from build123d import *

# Parameters (mm, degrees)
CROQUIS1_W               = 25
CROQUIS1_H               = 44
SALIENTE_EXTRUIR1_DEPTH  = 20
CROQUIS2_W               = 11.3
CROQUIS2_H               = 40.4
CORTAR_EXTRUIR1_DEPTH    = 18
CROQUIS3_W               = 10.7
CROQUIS3_H               = 44
CORTAR_EXTRUIR2_DEPTH    = 12
CORTAR_EXTRUIR3_START    = -25
CROQUIS4_R               = 1.6
CORTAR_EXTRUIR3_DEPTH    = 25
CROQUIS5_R               = 3
CORTAR_EXTRUIR4_DEPTH    = 17
CROQUIS7_W               = 10.7
CROQUIS7_H               = 2.131966011
SALIENTE_EXTRUIR2_DEPTH  = 12
CROQUIS9_W               = 11.3
CROQUIS9_H               = 12.16552506
SALIENTE_EXTRUIR3_DEPTH  = 2
SALIENTE_EXTRUIR4_DEPTH  = 2
CORTAR_EXTRUIR10_START   = -25
CROQUIS12_W              = 0.99
CROQUIS12_H              = 44
CORTAR_EXTRUIR10_DEPTH   = 25
CROQUIS13_W              = 8
CROQUIS13_H              = 44
CORTAR_EXTRUIR11_DEPTH   = 11.7
SALIENTE_EXTRUIR5_DEPTH  = 11.7
CROQUIS15_W              = 10.763613753
CROQUIS15_H              = 40.736067978
CORTAR_EXTRUIR12_DEPTH   = 4
CROQUIS16_R              = 1.5
SALIENTE_EXTRUIR6_DEPTH  = 1.2
CORTAR_EXTRUIR13_START   = -44
CORTAR_EXTRUIR13_DEPTH   = 44
CROQUIS18_W              = 0.936386247
CROQUIS18_H              = 40.568033989
CORTAR_EXTRUIR14_DEPTH   = 4
SALIENTE_EXTRUIR7_START  = -9.2
SALIENTE_EXTRUIR7_DEPTH  = 9.2
SALIENTE_EXTRUIR8_START  = -12.9
CROQUIS20_W              = 4
CROQUIS20_H              = 0.236067978
CROQUIS20_H_2            = 0.25
SALIENTE_EXTRUIR8_DEPTH  = 12.9
CROQUIS21_W              = 4
CROQUIS21_H              = 6.401046148
CROQUIS21_H_2            = 6.387114126
SALIENTE_EXTRUIR9_DEPTH  = 1.5
SALIENTE_EXTRUIR10_DEPTH = 0.4
CORTAR_EXTRUIR15_START   = -18
CROQUIS23_W              = 12.2
CROQUIS23_H              = 40.9
CORTAR_EXTRUIR15_DEPTH   = 18


with BuildPart() as part:
    # Croquis1 → Saliente-Extruir1 (new body)
    with BuildSketch(Plane.XY):
        with Locations((-22.114132301, -13.090425532)):
            Rectangle(CROQUIS1_W, CROQUIS1_H)
    extrude(amount=SALIENTE_EXTRUIR1_DEPTH)

    # Croquis2 → Cortar-Extruir1 (cut)
    with BuildSketch(Plane.XY.offset(20)):
        with Locations((-26.964132301, -13.090425532)):
            Rectangle(CROQUIS2_W, CROQUIS2_H)
    extrude(amount=-CORTAR_EXTRUIR1_DEPTH, mode=Mode.SUBTRACT)

    # Croquis3 → Cortar-Extruir2 (cut)
    with BuildSketch(Plane.XY.offset(20)):
        with Locations((-14.964132301, -13.090425532)):
            Rectangle(CROQUIS3_W, CROQUIS3_H)
    extrude(amount=-CORTAR_EXTRUIR2_DEPTH, mode=Mode.SUBTRACT)

    # Croquis4 → Cortar-Extruir3 (cut)
    with BuildSketch(Plane.ZY.offset(34.614132301).offset(CORTAR_EXTRUIR3_START)):
        with Locations((6, 2.409574468)):
            Circle(CROQUIS4_R)
        with Locations((6, -28.590425532)):
            Circle(CROQUIS4_R)
        with BuildLine():
            Line((20, 5.909574468), (20, -32.090425532))
            ThreePointArc((20, -32.090425532), (1, -13.090425532), (20, 5.909574468))
        make_face()
    extrude(amount=CORTAR_EXTRUIR3_DEPTH, mode=Mode.SUBTRACT)

    # Croquis5 → Cortar-Extruir4 (cut)
    with BuildSketch(Plane.ZY.offset(34.614132301)):
        with Locations((6, 2.409574468)):
            Circle(CROQUIS5_R)
        with Locations((6, -28.590425532)):
            Circle(CROQUIS5_R)
    extrude(amount=-CORTAR_EXTRUIR4_DEPTH, mode=Mode.SUBTRACT)

    # Croquis7 → Saliente-Extruir2 (add)
    with BuildSketch(Plane.XY.offset(8)):
        with Locations((-14.964132301, -34.024442527)):
            Rectangle(CROQUIS7_W, CROQUIS7_H)
        with Locations((-14.964132301, 7.843591463)):
            Rectangle(CROQUIS7_W, CROQUIS7_H)
    extrude(amount=SALIENTE_EXTRUIR2_DEPTH)

    # Croquis9 → Saliente-Extruir3 (add)
    with BuildSketch(Plane.XY.offset(2)):
        with Locations((-26.964132301, -13.090425532)):
            Rectangle(CROQUIS9_W, CROQUIS9_H)
    extrude(amount=-SALIENTE_EXTRUIR3_DEPTH)

    # Croquis11 → Saliente-Extruir4 (add)
    with BuildSketch(Plane.ZY.offset(32.614132301)):
        with BuildLine():
            Line((2, -7.007663002), (2, -19.173188062))
            ThreePointArc((2, -19.173188062), (1, -13.090425532), (2, -7.007663002))
        make_face()
    extrude(amount=SALIENTE_EXTRUIR4_DEPTH)

    # Croquis12 → Cortar-Extruir10 (cut)
    with BuildSketch(Plane.ZY.offset(34.614132301).offset(CORTAR_EXTRUIR10_START)):
        with Locations((0.495, -13.090425532)):
            Rectangle(CROQUIS12_W, CROQUIS12_H)
    extrude(amount=CORTAR_EXTRUIR10_DEPTH, mode=Mode.SUBTRACT)

    # Croquis13 → Cortar-Extruir11 (cut)
    with BuildSketch(Plane(origin=(-9.614132301, 0, 0), x_dir=(0, 0, -1), z_dir=(1, 0, 0))):
        with Locations((-16, -13.090425532)):
            Rectangle(CROQUIS13_W, CROQUIS13_H)
    extrude(amount=-CORTAR_EXTRUIR11_DEPTH, mode=Mode.SUBTRACT)

    # Croquis14 → Saliente-Extruir5 (add)
    with BuildSketch(Plane(origin=(-21.314132301, 0, 0), x_dir=(0, 0, -1), z_dir=(1, 0, 0))):
        with BuildLine():
            Line((-2, -19.173188062), (-2, -7.007663002))
            ThreePointArc((-2, -7.007663002), (-1, -13.090425532), (-2, -19.173188062))
        make_face()
    extrude(amount=SALIENTE_EXTRUIR5_DEPTH)

    # Croquis15 → Cortar-Extruir12 (cut)
    with BuildSketch(Plane.XY.offset(12)):
        with Locations((-14.995939178, -13.090425532)):
            Rectangle(CROQUIS15_W, CROQUIS15_H)
    extrude(amount=-CORTAR_EXTRUIR12_DEPTH, mode=Mode.SUBTRACT)

    # Croquis16 → Saliente-Extruir6 (add)
    with BuildSketch(Plane(origin=(-9.614132301, 0, 0), x_dir=(0, 0, -1), z_dir=(1, 0, 0))):
        with BuildLine():
            Line((-8, -27.821345395), (-8, -33.458459521))
            Line((-8, -33.458459521), (-12, -33.458459521))
            Line((-12, -33.458459521), (-12, -35.090425532))
            Line((-12, -35.090425532), (-0.99, -35.090425532))
            Line((-0.99, -35.090425532), (-0.99, 8.909574468))
            Line((-0.99, 8.909574468), (-12, 8.909574468))
            Line((-12, 8.909574468), (-12, 7.277608457))
            Line((-12, 7.277608457), (-8, 7.277608457))
            Line((-8, 7.277608457), (-8, 1.640494331))
            ThreePointArc((-8, 1.640494331), (-4.389181434, -2.259804881), (-2, -7.007663002))
            Line((-2, -7.007663002), (-2, -19.173188062))
            ThreePointArc((-2, -19.173188062), (-4.389181434, -23.921046183), (-8, -27.821345395))
        make_face()
        with Locations((-6, -28.590425532)):
            Circle(CROQUIS16_R, mode=Mode.SUBTRACT)
        with Locations((-6, 2.409574468)):
            Circle(CROQUIS16_R, mode=Mode.SUBTRACT)
    extrude(amount=SALIENTE_EXTRUIR6_DEPTH)

    # Croquis17 → Cortar-Extruir13 (cut)
    with BuildSketch(Plane.XZ.offset(35.090425532).offset(CORTAR_EXTRUIR13_START)):
        Polygon((-21.314132301, 12), (-21.314132301, 20), (-27.964132301, 20), align=None)
    extrude(amount=CORTAR_EXTRUIR13_DEPTH, mode=Mode.SUBTRACT)

    # Croquis18 → Cortar-Extruir14 (cut)
    with BuildSketch(Plane.XY.offset(12)):
        with Locations((-20.845939178, -13.006408538)):
            Rectangle(CROQUIS18_W, CROQUIS18_H)
    extrude(amount=-CORTAR_EXTRUIR14_DEPTH, mode=Mode.SUBTRACT)

    # Croquis19 → Saliente-Extruir7 (add)
    with BuildSketch(Plane(origin=(-8.414132301, 0, 0), x_dir=(0, 0, -1), z_dir=(1, 0, 0)).offset(SALIENTE_EXTRUIR7_START)):
        with BuildLine():
            Line((-2, -19.173188062), (-2, -7.007663002))
            ThreePointArc((-2, -7.007663002), (-4.389181434, -2.259804881), (-8, 1.640494331))
            Line((-8, 1.640494331), (-8, 0.640494331))
            ThreePointArc((-8, 0.640494331), (-5.026875227, -2.874277954), (-3, -7.007663002))
            Line((-3, -7.007663002), (-3, -19.173188062))
            ThreePointArc((-3, -19.173188062), (-4.972698099, -23.341991528), (-8, -26.821345395))
            Line((-8, -26.821345395), (-8, -27.821345395))
            ThreePointArc((-8, -27.821345395), (-4.389181434, -23.921046183), (-2, -19.173188062))
        make_face()
    extrude(amount=SALIENTE_EXTRUIR7_DEPTH)

    # Croquis20 → Saliente-Extruir8 (add)
    with BuildSketch(Plane(origin=(-8.414132301, 0, 0), x_dir=(0, 0, -1), z_dir=(1, 0, 0)).offset(SALIENTE_EXTRUIR8_START)):
        with Locations((-10, -33.340425532)):
            Rectangle(CROQUIS20_W, CROQUIS20_H)
        with Locations((-10, 7.152608457)):
            Rectangle(CROQUIS20_W, CROQUIS20_H_2)
    extrude(amount=SALIENTE_EXTRUIR8_DEPTH)

    # Croquis21 → Saliente-Extruir9 (add)
    with BuildSketch(Plane(origin=(-8.414132301, 0, 0), x_dir=(0, 0, -1), z_dir=(1, 0, 0))):
        with Locations((-10, -30.021868469)):
            Rectangle(CROQUIS21_W, CROQUIS21_H)
        with Locations((-10, 3.834051394)):
            Rectangle(CROQUIS21_W, CROQUIS21_H_2)
    extrude(amount=-SALIENTE_EXTRUIR9_DEPTH)

    # Croquis22 → Saliente-Extruir10 (add)
    with BuildSketch(Plane.XY.offset(8)):
        Polygon((-9.914132301, 7.027608457), (-21.314132301, 7.027608457), (-21.314132301, 4.645642446), (-17.614132301, 4.645642446), (-17.614132301, 0.640494331), (-9.914132301, 0.640494331), align=None)
        Polygon((-9.914132301, -26.821345395), (-17.614132301, -26.821345395), (-17.614132301, -30.826493509), (-21.314132301, -30.826493509), (-21.314132301, -33.222391543), (-9.914132301, -33.222391543), align=None)
    extrude(amount=SALIENTE_EXTRUIR10_DEPTH)

    # Croquis23 → Cortar-Extruir15 (cut)
    with BuildSketch(Plane.XY.offset(20).offset(CORTAR_EXTRUIR15_START)):
        with Locations((-27.014132301, -13.090425532)):
            Rectangle(CROQUIS23_W, CROQUIS23_H)
    extrude(amount=CORTAR_EXTRUIR15_DEPTH, mode=Mode.SUBTRACT)


solid = part.part
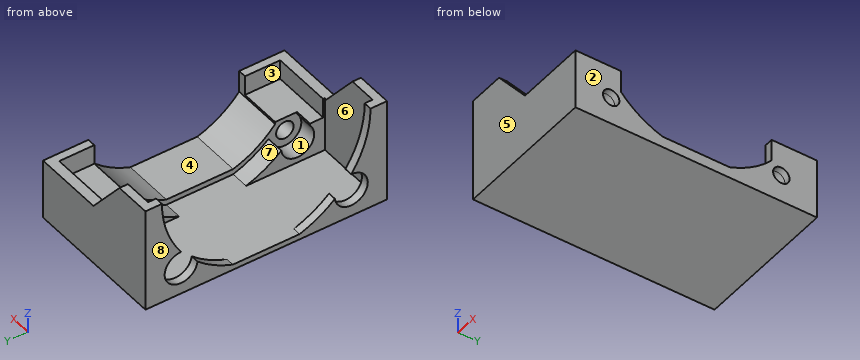
Source: CAD feature listing. Evaluate the final solid. Frame: model axes, mm. Face numbers are marked on the shaded views. A direction names the side the tool comes from. Coordinates: 2 decimals unless noted, no trailing zeros. Loops run counter-clockwise (first coordinate to the right, second up) from the corner with the lowest first, then second, coordinate; pieces in that order, holes last. Notation, with made-up numbers: (21.25, 12.5) -> (43.25, 12.5) arc R37 cw to (43.25, 49.5) -> close; hole circle Ø4 at (17, -22.5). An arc over 180 degrees is marked (long way). Answer in a Markdown table with one row per item. Add a question column.
Q1. Section D-D on y = -4. Return the cut outline in (x, z).
Q2. Pull-direction query (X, two-part tool) for the marked faces 6, 7 and 8; classes: pulls with the +X half, pulls with the -X half, needs draft (parallel to the pull), parting line crosses it, or undercut.
Q3. Section C-C on x = -22.5. Return the cut outline in (y, z).
Q4. Ray query, line 1 along X through (y, z) = (6.5, 7); line 2 along Y through (x, z) = (-26.25, 11); line 3 along Y through (x, z) = (-34.1, 6). Return the intervals inside material, ascending.
Q5. Section A-A on z = 13. Return the cut outline in (x, y).
Q6. Contact query for flat-ended pins moving along their axis: pin 1 Ø8 at (y, z) = (-1.5, 9) entering from -X; pin 2 Ø3 at (x, y) = (-14.5, -5) entering from +Z; pin 3 Ø4.5 at (x, y) = (-14.5, -12.5) entering from +Z; pin 4 Ø1.9 at (x, y) = (-15.5, 3.5) entering from +Z. Output: stop coordinate, or through.
Q7. Section B-B on x = -11.25. Return the cut outline in (y, z), and give its area (3 significant figures).
Q8. Reachability of the marked faces 1, 2, 3, 4 and 5 from +Z, -Z, +X, -X, +Y, -Y: full face, straight path, thin tool, end or side. Return the list, or none.
Computed values:
| question | item | result |
|---|---|---|
| 1 | outline | (-34.61, 0.99) -> (-8.41, 0.99) -> (-8.41, 4.35) -> (-17.61, 4.35) -> (-17.61, 3.32) -> (-20.91, 3.32) -> (-20.91, 2) -> (-33.11, 2) -> (-33.11, 3.32) -> (-34.61, 3.32) -> close |
| 2 | face 6 | undercut |
| 2 | face 7 | needs draft |
| 2 | face 8 | pulls with the -X half |
| 3 | outline | (-35.09, 0.99) -> (8.91, 0.99) -> (8.91, 13.43) -> (7.36, 13.43) -> (7.36, 2) -> (-33.54, 2) -> (-33.54, 13.43) -> (-35.09, 13.43) -> close |
| 4 | line 1 | x = -34.61 to -33.11, -20.91 to -8.41 |
| 4 | line 2 | y = -35.09 to -33.54, 7.36 to 8.91 |
| 4 | line 3 | y = -35.09 to -31.59, 5.41 to 8.91 |
| 5 | outline | (-34.61, -35.09) -> (-22.15, -35.09) -> (-22.15, -33.54) -> (-33.11, -33.54) -> (-33.11, -30.75) -> (-34.61, -30.75) -> close; (-34.61, 4.57) -> (-33.11, 4.57) -> (-33.11, 7.36) -> (-22.15, 7.36) -> (-22.15, 8.91) -> (-34.61, 8.91) -> close |
| 6 | pin 1 | stops at x = -34.61 |
| 6 | pin 2 | stops at z = 4.64 |
| 6 | pin 3 | stops at z = 3 |
| 6 | pin 4 | stops at z = 8.4 |
| 7 | outline | (-35.09, 0.99) -> (8.91, 0.99) -> (8.91, 12) -> (7.03, 12) -> (7.03, 8.4) -> (0.64, 8.4) -> (0.64, 8) arc R18.75 cw to (-7.01, 3) -> (-19.17, 3) arc R16.88 cw to (-26.82, 8) -> (-26.82, 8.4) -> (-33.22, 8.4) -> (-33.22, 12) -> (-35.09, 12) -> close; hole circle Ø3.2 at (-28.59, 6); hole circle Ø3.2 at (2.41, 6) |
| 7 | area | 206 mm^2 |
| 8 | face 1 | -X |
| 8 | face 2 | +Z, -Z, +X, +Y, -Y |
| 8 | face 3 | +Z |
| 8 | face 4 | +Z, +X, -X |
| 8 | face 5 | +Z, -Z, +X, -X, -Y |
